Input: part model. Units: mm. Frame: model coordinates. A direction names the side the tool comes from. Give positions to 0.01 mm unless a question says otherwise; leave off trailing zeros. Write each loop counter-clockwise with the first axis right and the second up, starting at its lowest first coordinate (ties: lowest second). Pieces come first, ordered by that corner, then holes.
```python
from build123d import *

# Parameters (mm, degrees)
F1_DEPTH = 1
F2_D     = 3
F2_DEPTH = 5
F2_TIP   = 0.9012909285
F3_W     = 2
F3_H     = 2
F4_DEPTH = 1
F5_W     = 9
F5_H     = 3
F6_DEPTH = 3
F7_W     = 2.5
F7_H     = 2.5
F8_DEPTH = 1


with BuildPart() as f1:
    # F0 (on Top) → F1 (new body)
    with BuildSketch(Plane.XY):
        with BuildLine():
            Line((12, 13.5), (-12, 13.5))
            ThreePointArc((-12, 13.5), (-13.0606601718, 13.0606601718), (-13.5, 12))
            Line((-13.5, 12), (-13.5, -12))
            ThreePointArc((-13.5, -12), (-13.0606601718, -13.0606601718), (-12, -13.5))
            Line((-12, -13.5), (12, -13.5))
            ThreePointArc((12, -13.5), (13.0606601718, -13.0606601718), (13.5, -12))
            Line((13.5, -12), (13.5, 12))
            ThreePointArc((13.5, 12), (13.0606601718, 13.0606601718), (12, 13.5))
        make_face()
    extrude(amount=-F1_DEPTH)

    # F2
    with Locations(Plane.XY):
        with Locations((-10, 10), (10, 10), (10, -10), (-10, -10)):
            Hole(F2_D / 2, depth=F2_DEPTH)
            with Locations((0, 0, -(F2_DEPTH + F2_TIP / 2))):  # 118° drill point
                Cone(0, F2_D / 2, F2_TIP, mode=Mode.SUBTRACT)

    # F3 (on face) → F4 (join)
    with BuildSketch(Plane(origin=(0, 0, -1), x_dir=(1, 0, 0), z_dir=(0, 0, -1))):
        with Locations((-14.5, 9.9446508034)):
            Rectangle(F3_W, F3_H)
        with Locations((-14.5, 5.9446508034)):
            Rectangle(F3_W, F3_H)
        with Locations((-14.5, 1.9446508034)):
            Rectangle(F3_W, F3_H)
        with Locations((-14.5, -2.0553491966)):
            Rectangle(F3_W, F3_H)
        with Locations((-14.5, -6.0553491966)):
            Rectangle(F3_W, F3_H)
        with Locations((-14.5, -10.0553491966)):
            Rectangle(F3_W, F3_H)
        with Locations((14.5, 9.9446508034)):
            Rectangle(F3_W, F3_H)
        with Locations((14.5, 5.9446508034)):
            Rectangle(F3_W, F3_H)
        with Locations((14.5, 1.9446508034)):
            Rectangle(F3_W, F3_H)
        with Locations((14.5, -2.0553491966)):
            Rectangle(F3_W, F3_H)
        with Locations((14.5, -6.0553491966)):
            Rectangle(F3_W, F3_H)
        with Locations((14.5, -10.0553491966)):
            Rectangle(F3_W, F3_H)
        with Locations((-2.5, -14.5)):
            Rectangle(F3_W, F3_H)
        with Locations((2.5, -14.5)):
            Rectangle(F3_W, F3_H)
    extrude(amount=-F4_DEPTH)

    # F5 (on face) → F6 (join)
    with BuildSketch(Plane.XY):
        with Locations((0, 12)):
            Rectangle(F5_W, F5_H)
    extrude(amount=F6_DEPTH)

    # F7 (on face) → F8 (join)
    with BuildSketch(Plane.XY):
        with Locations((-10.7858264819, 2.4961141907)):
            Rectangle(F7_W, F7_H)
        with Locations((-10.7858264819, -1.5038858093)):
            Rectangle(F7_W, F7_H)
        with Locations((-10.7858264819, -5.5038858093)):
            Rectangle(F7_W, F7_H)
        with Locations((-10.7858264819, 6.4961141907)):
            Rectangle(F7_W, F7_H)
        with Locations((10.2141735181, 6.4961141907)):
            Rectangle(F7_W, F7_H)
        with Locations((10.2141735181, 2.4961141907)):
            Rectangle(F7_W, F7_H)
        with Locations((10.2141735181, -1.5038858093)):
            Rectangle(F7_W, F7_H)
        with Locations((10.2141735181, -5.5038858093)):
            Rectangle(F7_W, F7_H)
    extrude(amount=F8_DEPTH)


solid = f1.part
```
Item 1: Section D-D (z = 0.55). Give the number of separate pieces and of enclosed holes in the cut face, and give its area (3 significant figures).
Item 2: Ray query, line 1 (Y direction, x = -10, z = -0.45); line 2 (X direction, y = -6, z = 0.1); line 3 (X direction, y = 9.75, z = -0.05). Return the intervals inside material, ascending.
Item 3: Set-up query: faces 1 (the flat face through (-13.5, 0.1, -0.5)), 2 (the flat face through (14.5, -4.945, -0.5)), 3 (the flat face through (-14.5, -10.945, -0.5)). Return all of +Z, -Z, +X, -X, +Y, -Y with unobstructed straight access to the full face (end or side cutting, diameter ignored); none if empty.
Item 4: Mould query, pull axis X, two halves, no side actions, for faces 4 (the flat face through (-15.5, 2.1, -0.5)), 5 (the flat face through (-11, -1, 1)), 6 (the cylindrical face through (-8.8, -10.9, -0.5)), 7 (the cylindrical face through (-8.8, 9.1, -0.5)). Classes: +X half, -X half, draft (parallel to the pull), parting line (faces both ways), or undercut.
Item 5: Pin query (flat end, axial travel): pin 1 (1.1 mm diameter, centred on x = 10.5, z = 0.5, fed in from -Y); pin 2 (0.5 mm diameter, centred on y = 2.5, z = 0.5, fed in from -X); pin 3 (0.8 mm diameter, centred on x = 9.5, z = 0.5, fed in from +Y); pin 4 (1.2 mm diameter, centred on x = 9.5, y = -2, fed in from +Z). Return the tip coordinate at first contact, or that it passes through.
Item 6: Section B-B (y = -10). Return loops of the section in (x, z), and give its area (3 significant figures).
Item 7: Section C-C (y = 6.25). Return loops of the section in (x, z), and give its area (3 significant figures).
Item 8: Section A-A (x = -10). Return loops of the section in (y, z), and give its area (3 significant figures).
Solved:
1. separate pieces: 9
1. enclosed holes: 0
1. area: 77.0 mm2
2. line 1: y = -13.5 to -11.5, -8.5 to 8.5, 11.5 to 13.5
2. line 2: x = -12.04 to -9.54, 8.96 to 11.46
2. line 3: x = -15.5 to -11.48, -8.52 to 8.52, 11.48 to 15.5
3. face 1: +Z, -Z, -X
3. face 2: +Z, -Z, +X
3. face 3: +Z, -Z, -X, -Y
4. face 4: -X half
4. face 5: draft
4. face 6: undercut
4. face 7: undercut
5. pin 1: stops at y = -13.5
5. pin 2: stops at x = -12.04
5. pin 3: stops at y = 7.75
5. pin 4: stops at z = 1
6. outline: (-15.5, -1) - (-11.5, -1) - (-11.5, 0) - (-15.5, 0) - close; (-8.5, -1) - (8.5, -1) - (8.5, 0) - (-8.5, 0) - close; (11.5, -1) - (15.5, -1) - (15.5, 0) - (11.5, 0) - close
6. area: 25.0 mm2
7. outline: (-15.5, -1) - (15.5, -1) - (15.5, 0) - (11.46, 0) - (11.46, 1) - (8.96, 1) - (8.96, 0) - (-9.54, 0) - (-9.54, 1) - (-12.04, 1) - (-12.04, 0) - (-15.5, 0) - close
7. area: 36.0 mm2
8. outline: (-13.5, -1) - (-11.5, -1) - (-11.5, 0) - (-13.5, 0) - close; (-8.5, -1) - (8.5, -1) - (8.5, 0) - (7.75, 0) - (7.75, 1) - (5.25, 1) - (5.25, 0) - (3.75, 0) - (3.75, 1) - (1.25, 1) - (1.25, 0) - (-0.25, 0) - (-0.25, 1) - (-2.75, 1) - (-2.75, 0) - (-4.25, 0) - (-4.25, 1) - (-6.75, 1) - (-6.75, 0) - (-8.5, 0) - close; (11.5, -1) - (13.5, -1) - (13.5, 0) - (11.5, 0) - close
8. area: 31.0 mm2
